from build123d import *

# Parameters (mm, degrees)
SKETCH1_W           = 129.8
SKETCH1_H           = 65
BOSS_EXTRUDE1_DEPTH = 9
SKETCH2_R           = 2.35
CUT_EXTRUDE1_DEPTH  = 8
CHAMFER1_SIZE       = 1
CHAMFER2_SIZE       = 9


with BuildPart() as part:
    # Sketch1 → Boss-Extrude1 (new body)
    with BuildSketch(Plane(origin=(0, 0, 0), x_dir=(1, 0, 0), z_dir=(0, 1, 0))):
        Rectangle(SKETCH1_W, SKETCH1_H)
    extrude(amount=BOSS_EXTRUDE1_DEPTH)

    # Sketch2 → Cut-Extrude1 (cut)
    with BuildSketch(Plane.XZ):
        with Locations(Location((-32.45, 20, 0), (0, 0, 270))):
            Circle(SKETCH2_R)
        with Locations(Location((0, 20, 0), (0, 0, 270))):
            Circle(SKETCH2_R)
        with Locations(Location((32.45, 20, 0), (0, 0, 270))):
            Circle(SKETCH2_R)
        with Locations(Location((32.45, -20, 0), (0, 0, 90))):
            Circle(SKETCH2_R)
        with Locations(Location((0, -20, 0), (0, 0, 90))):
            Circle(SKETCH2_R)
        with Locations(Location((-32.45, -20, 0), (0, 0, 90))):
            Circle(SKETCH2_R)
    extrude(amount=-CUT_EXTRUDE1_DEPTH, mode=Mode.SUBTRACT)

    # Chamfer1
    chamfer1_edges = [part.edges().sort_by_distance(p)[0] for p in [
        (-32.45, 0, -22.35),
        (0, 0, -22.35),
        (32.45, 0, -22.35),
        (32.45, 0, 22.35),
        (0, 0, 22.35),
        (-32.45, 0, 22.35),
    ]]
    chamfer(chamfer1_edges, length=CHAMFER1_SIZE)

    # Chamfer2
    chamfer2_edges = [part.edges().sort_by_distance(p)[0] for p in [
        (0, 9, 32.5),
        (0, 9, -32.5),
    ]]
    chamfer(chamfer2_edges, length=CHAMFER2_SIZE - 0.0001)  # a hair under: the kernel refuses the full size


solid = part.part
Read the model definition and answer for the solid it produces. Units are mm, in the model's axes. A direction names the side the tool comes from. Coordinates: 2 decimals unless noted, no trailing zeros. Order: outer loops, then holes, each group sorted by start corner. A loop starts at its lowest first (then second) coordinate and runs counter-clockwise, first axis right, second up. Notation, with made-up numbers: (60, 61) - (74, 61) arc R14 cw to (74, 68) - close; hole circle Ø11 at (39.25, 62.5). An arc over 180 degrees is marked (long way). Use one line per item in the form item = value.
(1) Straight lines are drawn through the part: L1, parallel to X at y = 3, z = -20; L2, parallel to X at y = 3.5, z = 21; L3, parallel to Z at x = -26, y = 3.75. For each, find the intervals that lie inside material, in ascending order.
Computed values:
L1 = -64.9 to -34.8, -30.1 to -2.35, 2.35 to 30.1, 34.8 to 64.9
L2 = -64.9 to -34.58, -30.32 to -2.13, 2.13 to 30.32, 34.58 to 64.9
L3 = -28.75 to 28.75
(2) Section B-B, the plane z = -20 is taken. Give the vertices of the cut face in (x, y), then the cut area to 3 significant figures.
Computed values:
outline = (-64.9, 0) - (-35.8, 0) - (-34.8, 1) - (-34.8, 8) - (-30.1, 8) - (-30.1, 1) - (-29.1, 0) - (-3.35, 0) - (-2.35, 1) - (-2.35, 8) - (2.35, 8) - (2.35, 1) - (3.35, 0) - (29.1, 0) - (30.1, 1) - (30.1, 8) - (34.8, 8) - (34.8, 1) - (35.8, 0) - (64.9, 0) - (64.9, 9) - (-64.9, 9) - close
area = 1,050 mm²
(3) Section C-C, the plane y = 5.5 is taken. Give the vertices of the cut face in (x, z).
Computed values:
outline = (-64.9, -27) - (64.9, -27) - (64.9, 27) - (-64.9, 27) - close; hole circle Ø4.7 at (-32.45, -20); hole circle Ø4.7 at (-32.45, 20); hole circle Ø4.7 at (0, -20); hole circle Ø4.7 at (0, 20); hole circle Ø4.7 at (32.45, -20); hole circle Ø4.7 at (32.45, 20)
(4) For a pull along X with two mould halves and no side action, classify faces 1 (the face through (34.04, 4.45, 21.73)), 2 (the face through (-64.9, 4, 0)), 3 (the face through (0.103, 4.451, 22.348)), 4 (the face through (-0.9, 4.6, -27.9)) as pulls with the +X half, pulls with the -X half, needs draft (parallel to the pull), parting line crosses it, or undercut.
Computed values:
face_1 = undercut
face_2 = pulls with the -X half
face_3 = undercut
face_4 = needs draft
(5) Which of the six approach directions +Z, -Z, +X, -X, +Y, -Y give full straight-line access (tool end or side, diameter ignored) to faces 5 (the face through (-1, 9, 0)), 6 (the face through (0, 8, -20))?
Computed values:
face_5 = +Z, -Z, +X, -X, +Y
face_6 = -Y
(6) Given pin 1 Ø5 at (x, y) = (35, 6.5) entering from +Z; pin 2 Ø5 at (x, y) = (-12, 4.5) entering from -Z; pin 3 Ø5 at (x, z) = (31.5, -21) entering from -Y; pin 4 Ø2.5 at (x, z) = (-0.5, -20.5) entering from -Y, each flat-ended and moving along its own axis, determine where each tip first touches the part or whether it passes through.
Computed values:
pin_1 = 28.5
pin_2 = -30.5
pin_3 = 0
pin_4 = 8
